from build123d import *

# Parameters (mm, degrees)
PAD_DEPTH    = 3
POCKET_DEPTH = 3.001


with BuildPart() as part:
    # Sketch → Pad (new body)
    with BuildSketch(Plane.XY):
        with BuildLine():
            Line((-52.625, 23.225), (-52.625, -23.225))
            ThreePointArc((-52.625, -23.225), (-51.453427, -26.053427), (-48.625, -27.225))
            Line((-48.625, -27.225), (48.625, -27.225))
            ThreePointArc((48.625, -27.225), (51.453427, -26.053427), (52.625, -23.225))
            Line((52.625, -23.225), (52.625, 23.225))
            ThreePointArc((52.625, 23.225), (51.453427, 26.053427), (48.625, 27.225))
            Line((48.625, 27.225), (-48.625, 27.225))
            ThreePointArc((-48.625, 27.225), (-51.453427, 26.053427), (-52.625, 23.225))
        make_face()
    extrude(amount=PAD_DEPTH)

    # Sketch001 (on Face10 of Pad) → Pocket (cut, through all)
    with BuildSketch(Plane.XY.offset(3)):
        Polygon((-44.853719, -22.225), (-46.239359, -19.825), (-49.010641, -19.825), (-50.396281, -22.225), (-49.010641, -24.625), (-46.239359, -24.625), align=None)
        Polygon((44.853719, -22.225), (46.239359, -24.625), (49.010641, -24.625), (50.396281, -22.225), (49.010641, -19.825), (46.239359, -19.825), align=None)
        Polygon((44.853719, 22.225), (46.239359, 19.825), (49.010641, 19.825), (50.396281, 22.225), (49.010641, 24.625), (46.239359, 24.625), align=None)
        Polygon((-44.853719, 22.225), (-46.239359, 24.625), (-49.010641, 24.625), (-50.396281, 22.225), (-49.010641, 19.825), (-46.239359, 19.825), align=None)
    extrude(amount=-POCKET_DEPTH, mode=Mode.SUBTRACT)


solid = part.part
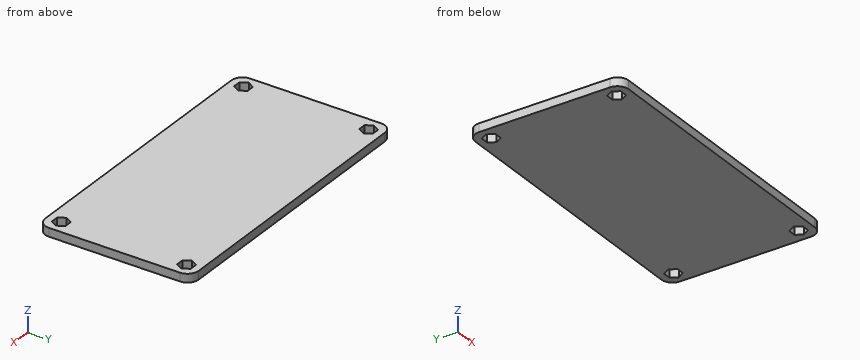
Read the model definition and answer for the solid it produces. Units are mm, in the model's axes. Coordinates: 2 decimals unless noted, no trailing zeros. Order: outer loops, then holes, each group sorted by start corner. A loop starts at its lowest first (then second) coordinate and runs counter-clockwise, first axis right, second up. Notation, with made-up numbers: (11, -3.75) - (57, -3.75) arc R16 cw to (57, 17.25) - close; hole circle Ø4 at (35.25, 76). An arc over 180 degrees is marked (long way). Use one line per item in the form item = value.
(1) Section B-B, the plane y = 21 is taken. Give the vertices of the cut face in (x, z) (3 decimals).
Computed values:
outline = (-52.625, 0) - (-49.689, 0) - (-49.689, 3) - (-52.625, 3) - close; (-45.561, 0) - (45.561, 0) - (45.561, 3) - (-45.561, 3) - close; (49.689, 0) - (52.625, 0) - (52.625, 3) - (49.689, 3) - close
(2) Straight lines are drawn through the part: L1, parallel to X at y = -23, z = 1.8 (3 decimals); L2, parallel to X at y = 24.5, z = 2.1; L3, parallel to Y at x = -46, z = 1.8 (3 decimals). For each, find the intervals that lie inside material, in ascending order.
Computed values:
L1 = -52.625 to -49.949, -45.301 to 45.301, 49.949 to 52.625
L2 = -52.42 to -49.08, -46.17 to 46.17, 49.08 to 52.42
L3 = -27.225 to -24.21, -20.24 to 20.24, 24.21 to 27.225
(3) Section A-A, the plane z = 0.7 is taken. Give the number of separate pieces and of enclosed holes in the cut face, then the cut area to 3 significant figures.
Computed values:
separate_pieces = 1
enclosed_holes = 4
area = 5,640 mm²
